Can you work these out from the model? Positions are in its coordinate system, mm. Face numbers are marked on the shaded views. A direction names the side the tool comes from. Round coordinates to 2 decimals unless told otherwise and drop trailing zeros. Write each loop counter-clockwise with the first axis right and the second up, starting at its lowest first coordinate (ties: lowest second). Pieces come first, ordered by that corner, then holes. Notation, with made-up numbers: (-1, -37) -> (49, -37) arc R27 ccw to (49, -17) -> close; hole circle Ø8 at (40.25, 81). An arc over 180 degrees is marked (long way). Write item = value, one per line. Start each with the question number.
1) If I drill on line 1 (X direction, y = 1.1, z = -5); line 2 (Z direction, x = 0, y = 1); line 3 (X direction, y = 14, z = -13), over which ranges is the centre line in solid material (lowest first)?
2) Imagine slicing it at B-B, the plane z = -5. Please give me the cut outline in (x, y).
3) Imagine slicing it at C-C, the plane y = 1.25. Please give me the cut outline in (x, z), then the cut area to 3 significant figures.
4) Thinking about a two-plate mould opening in Z: for the marked faces 4, 5, 6 and 7, which applies, +Z half, -Z half, draft (parallel to the pull), parting line (faces both ways), or undercut?
5) For the marked faces 1, 2 and 3, which set-ups out of +Z, -Z, +X, -X, +Y, -Y let a thin tool reach every point of the face, with its end or its side?
6) I'm going to push flat-ended pins straight in: pin 1 (1.2 mm diameter, centred on x = 3, y = 9.5, fed in from +Z); pin 2 (1.2 mm diameter, centred on x = -4, y = 10.5, fed in from -Z); pin 3 (1.5 mm diameter, centred on y = 4, z = -7.5, fed in from -X); pin 4 (1.5 mm diameter, centred on x = 4.5, z = 3, fed in from +Y). Where does each tip first touch, or does it pass through?
7) Imagine slicing it at A-A, the plane x = 0. Please give me the cut outline in (y, z).
8) Imagine slicing it at D-D, the plane x = -4.75. Please give me the cut outline in (y, z).
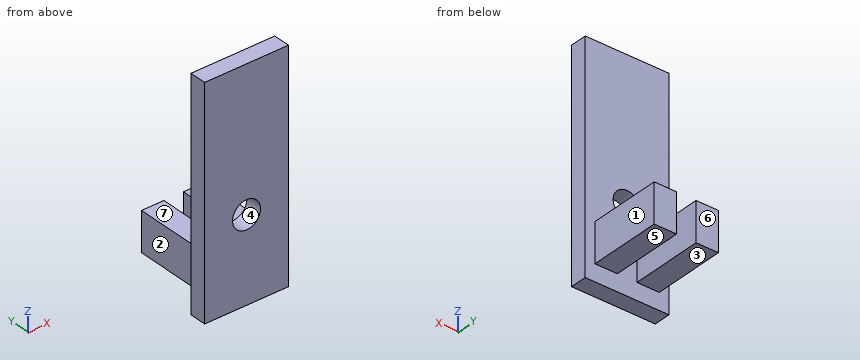
Autodesk Inventor part; units mm, degrees
ref_plane "YZ Plane" through (0, 0, 0) normal (1, 0, 0) x (0, 1, 0)
ref_plane "XZ Plane" through (0, 0, 0) normal (0, 1, 0) x (-1, 0, 0)
ref_plane "XY Plane" through (0, 0, 0) normal (0, 0, 1) x (1, 0, 0)
sketch "Sketch1" plane through (0, 0, 0) normal (0, 1, 0) x (-1, 0, 0)
  line L0 (7.5, 20) -> (-7.5, 20)
  line L1 (-7.5, 20) -> (-7.5, -20)
  line L2 (-7.5, -20) -> (7.5, -20)
  line L3 (7.5, -20) -> (7.5, 20)
  line L4 (7.5, 20) -> (-7.5, -20) construction
  line L5 (-7.5, 20) -> (7.5, -20) construction
  point P0 (0, 0)
  dimension "d0" = 15
  dimension "d1" = 40
extrude "Extrusion1" add sketch "Sketch1" along normal blind 3
sketch "Sketch2" plane through (0, 3, 0) normal (0, 1, 0) x (1, 0, 0)
  line L0 (0, 0) -> (0, 5)
  circle A0 centre (0, 5) radius 2.5
  line L1 (0, 5) -> (0, 10)
  line L2 (0, 10) -> (-3.75, 10)
  line L3 (-3.75, 10) -> (-3.75, 13.5)
  line L4 (-5.75, 10) -> (-1.75, 10)
  line L5 (-1.75, 10) -> (-1.75, 17)
  line L6 (-1.75, 17) -> (-5.75, 17)
  line L7 (-5.75, 17) -> (-5.75, 10)
  line L8 (-5.75, 10) -> (-1.75, 17) construction
  line L9 (-1.75, 10) -> (-5.75, 17) construction
  line L10 (3.75, 10) -> (3.75, 13.5)
  line L11 (5.75, 10) -> (1.75, 10)
  line L12 (1.75, 10) -> (1.75, 17)
  line L13 (1.75, 17) -> (5.75, 17)
  line L14 (5.75, 17) -> (5.75, 10)
  line L15 (5.75, 10) -> (1.75, 17) construction
  line L16 (1.75, 10) -> (5.75, 17) construction
  dimension "d4" = 5
  dimension "d5" = 5
  dimension "d6" = 5
  dimension "d7" = 3.75
  dimension "d8" = 3.5
  dimension "d9" = 4
  dimension "d10" = 7
extrude "Extrusion2" add sketch "Sketch2" along normal blind 13 contours L2 L4 L7 L6 L5 | L11 L12 L13 L14
extrude "Extrusion3" cut sketch "Sketch2" against normal blind 13 contours A0 L1 L0 | L0 L1 A0
properties part number "KY 032 INFRERROJO"
Reported:
q1.line_1 = -7.5 to -2.5, 2.5 to 7.5
q1.line_2 = -20 to -7.5, -2.5 to 20
q1.line_3 = -5.75 to -1.75, 1.75 to 5.75
q2.outline = (-7.5, 0) -> (-2.5, 0) -> (-2.5, 3) -> (-7.5, 3) -> close; (2.5, 0) -> (7.5, 0) -> (7.5, 3) -> (2.5, 3) -> close
q3.outline = (-7.5, -20) -> (7.5, -20) -> (7.5, 20) -> (-7.5, 20) -> close; hole circle Ø5 at (0, -5)
q3.area = 580 mm²
q4.face_4 = undercut
q4.face_5 = -Z half
q4.face_6 = draft
q4.face_7 = +Z half
q5.face_1 = +Z, -Z, +X, +Y
q5.face_2 = +Z, -Z, -X, +Y
q5.face_3 = -Z, +X, -X, +Y
q6.pin_1 = -10
q6.pin_2 = -17
q6.pin_3 = through
q6.pin_4 = 3
q7.outline = (0, -20) -> (3, -20) -> (3, -7.5) -> (0, -7.5) -> close; (0, -2.5) -> (3, -2.5) -> (3, 20) -> (0, 20) -> close
q8.outline = (0, -20) -> (3, -20) -> (3, -17) -> (16, -17) -> (16, -10) -> (3, -10) -> (3, 20) -> (0, 20) -> close
